Autodesk Inventor part; units mm, degrees
ref_plane "Work Plane1" through (-24.5, -7, 2.5) normal (0, 0, 1) x (1, 0, 0)
ref_plane "Work Plane2" through (-24.5, 2, 40.5) normal (0, -1, 0) x (1, 0, 0)
ref_plane "YZ Plane" through (0, 0, 0) normal (1, 0, 0) x (0, 1, 0)
sketch "Sketch2" plane through (0, 0, 0) normal (0, 0, 1) x (1, 0, 0)
  line L0 (-24.5, 0) -> (-24.5, 7)
  line L1 (-24.5, 0) -> (-24.5, -7)
  line L2 (-24.5, 7) -> (-19.799, 7)
  line L3 (-24.5, -7) -> (-19.799, -7)
  line L4 (24.5, 7) -> (19.799, 7)
  line L5 (24.5, 0) -> (24.5, 7)
  line L6 (24.5, 0) -> (24.5, -7)
  line L7 (24.5, -7) -> (19.799, -7)
  arc A0 (-19.799, -7) -> (19.799, -7) centre (0, 0) ccw
  arc A1 (19.799, 7) -> (-19.799, 7) centre (0, 0) ccw
  circle A2 centre (0, 0) radius 2.75
  point P0 (0, 0)
  point P1 (0, -4.75)
  point P2 (-27.5, 17.25)
  dimension "d0" = 5.5
extrude "Extrusion1" add sketch "Sketch2" along normal blind 2.5
ref_plane "Work Plane1" through (-24.5, -7, 2.5) normal (0, 0, 1) x (1, 0, 0)
sketch "Sketch3" plane through (-24.5, -7, 2.5) normal (0, 0, 1) x (1, 0, 0)
  line L0 (0, 14) -> (49, 14)
  line L1 (49, 14) -> (49, 9)
  line L2 (49, 9) -> (0, 9)
  line L3 (0, 9) -> (0, 14)
  dimension "d3" = 5
extrude "Extrusion2" add sketch "Sketch3" along normal blind 38
ref_plane "Work Plane2" through (-24.5, 2, 40.5) normal (0, -1, 0) x (1, 0, 0)
sketch "Sketch6" plane through (-24.5, 2, 40.5) normal (0, -1, 0) x (1, 0, 0)
  line L0 (0, -40.5) -> (0, -38)
  line L1 (-8.6, 0) -> (0, 0)
  line L2 (0, 0) -> (0, -38)
  arc A0 (-8.6, 0) -> (-14.3279, -9.2551) centre (-8.6, -6.4) ccw
  line L3 (0, -38) -> (-14.3279, -9.2551)
  line L4 (49, -40.5) -> (49, 0)
  arc A1 (63.3279, -9.2551) -> (57.6, 0) centre (57.6, -6.4) ccw
  line L5 (0, 0) -> (49, 0)
  line L6 (49, 0) -> (57.6, 0)
  line L7 (49, -38) -> (63.3279, -9.2551)
  point P0 (24.5, -40.5)
extrude "Extrusion5" add sketch "Sketch6" against normal blind 5
sketch "Sketch7" plane through (-24.5, 2, 40.5) normal (0, -1, 0) x (1, 0, 0)
  line L0 (24.5, -6.5) -> (116.5, -6.5) construction
  line L1 (15.25, 85.5) -> (-8.6, 0)
  line L2 (33.75, 85.5) -> (57.6, 0)
  line L3 (15.25, 85.5) -> (21.25, 85.5)
  line L4 (33.75, 85.5) -> (27.75, 85.5)
  line L5 (57.6, 0) -> (32.6, 0)
  line L6 (-8.6, 0) -> (16.4, 0)
  line L7 (21.25, 85.5) -> (16.4, 0)
  line L8 (27.75, 85.5) -> (32.6, 0)
  point P0 (24.5, -40.5)
sketch "Sketch8" plane through (-24.5, 2, 40.5) normal (0, -1, 0) x (1, 0, 0)
  circle A0 centre (24.5, -6.519) radius 2.75
  point P0 (24.5, -40.5)
  dimension "d35" = 5.5
extrude "Extrusion6" add sketch "Sketch7" against normal blind 5
extrude "Extrusion7" cut sketch "Sketch8" against normal blind 5
properties part number "gripper" material "ABS Plastic"
Part model, mm, in its own coordinate system. A direction names the side the tool comes from. Coordinates: 2 decimals unless noted, no trailing zeros. Write each loop counter-clockwise with the first axis right and the second up, starting at its lowest first coordinate (ties: lowest second). Pieces come first, ordered by that corner, then holes. Notation, with made-up numbers: M -1,-22.75 L 45,-22.75 A21 ccw 45,-11.75 Z; hole C 64,15.5 d2. An arc over 180 degrees is marked long. Return JSON: item names as keys, results as strings.
1. Saw through at D-D, the plane y = -14.5. Write the cut outline in (x, z), then the cut area to 3 significant figures.
Determined:
{"outline": "M -15.19,0 L 15.19,0 L 15.19,2.5 L -15.19,2.5 Z", "area": "76.0 mm²"}
2. Saw through at C-C, the plane z = 91. Write the cut outline in (x, y).
Determined:
{"outline": "M -19.01,2 L -5.24,2 L -5.24,7 L -19.01,7 Z; M 5.24,2 L 19.01,2 L 19.01,7 L 5.24,7 Z"}
3. Saw through at A-A, the plane y = 0. Write the cut outline in (x, z).
Determined:
{"outline": "M -24.5,0 L -2.75,0 L -2.75,2.5 L -24.5,2.5 Z; M 2.75,0 L 24.5,0 L 24.5,2.5 L 2.75,2.5 Z"}
4. Flat gauge pins, fed straight in: pin 1 Ø4 at (x, y) = (6, 14) entering from +Z; pin 2 Ø3 at (y, z) = (2.5, 1.5) entering from -X; pin 3 Ø3 at (x, z) = (22, 1) entering from -Y; pin 4 Ø3.5 at (x, z) = (0, 33.981) entering from -Y. Where does each tip first touch, or does it go through?
Determined:
{"pin 1": "z = 2.5", "pin 2": "x = -24.75", "pin 3": "y = -7", "pin 4": "through"}
5. 3-axis set-ups, long thin cutter, end or side, ignore diameter. For faces 1 (the face through (-0.596, 2.685, 1.232)), 2 (the face through (-24.5, 0, 1)), 3 (the face through (0, 13, 2.5)), 4 (the face through (-22, -7, 1)): which of +Z, -Z, +X, -X, +Y, -Y reach the whole face in a straight line?
Determined:
{"face 1": "-Z", "face 2": "-Z, -X, +Y, -Y", "face 3": "+Z, +X, -X, +Y", "face 4": "+Z, -Z, -X, -Y"}
6. Saw through at B-B, the plane x = 0. Write the cut outline in (y, z).
Determined:
{"outline": "M -21,0 L -2.75,0 L -2.75,2.5 L -21,2.5 Z; M 2,2.5 L 2.75,2.5 L 2.75,0 L 21,0 L 21,2.5 L 7,2.5 L 7,31.23 L 2,31.23 Z; M 2,36.73 L 7,36.73 L 7,40.5 L 2,40.5 Z"}
7. Pull direction X, two halves, no side cores. Call faces 5 (the face through (31.564, 4.465, 16.671)), 6 (the face through (0, -7, 2.5)), 7 (the face through (5.64, 4.46, 83.85)): pulls with the +X half, pulls with the -X half, needs draft (parallel to the pull), parting line crosses it, or undercut.
Determined:
{"face 5": "pulls with the +X half", "face 6": "needs draft", "face 7": "undercut"}
8. Probe L1, parallel to Y at x = 0, z = 1.3; L2, parallel to Z at x = 0, y = 5.8; L3, parallel to X at y = 0, z = 1. List the from-to ranges inside material, lowest first.
Determined:
{"L1": "-21 to -2.75, 2.75 to 21", "L2": "0 to 31.23, 36.73 to 40.5", "L3": "-24.5 to -2.75, 2.75 to 24.5"}
